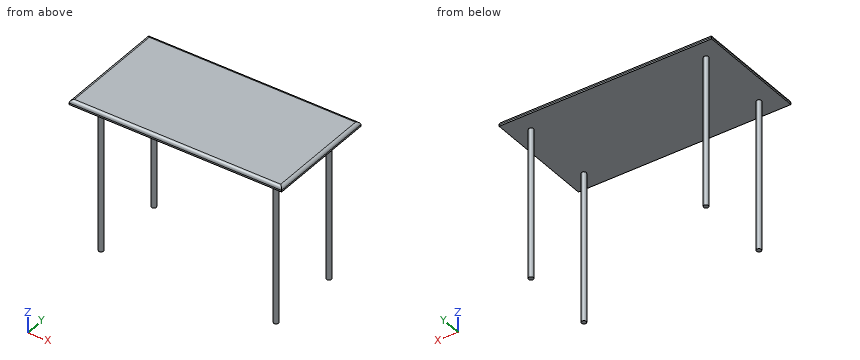
```python
from build123d import *

# Parameters (mm, degrees)
F0_R     = 9.525
F1_DEPTH = 609.6
F2_W     = 863.6
F2_H     = 457.2
F2_R     = 9.525
F3_DEPTH = 19.05
F4_R     = 12.7


with BuildPart() as f1:
    # F0 (on Top) → F1 (new body)
    with BuildSketch(Plane.XY):
        with Locations((9.933765, 11.337449)):
            Circle(F0_R)
        with Locations((9.933765, 316.137449)):
            Circle(F0_R)
        with Locations((721.133765, 11.337449)):
            Circle(F0_R)
        with Locations((721.133765, 316.137449)):
            Circle(F0_R)
    extrude(amount=F1_DEPTH)

    # F2 (on face) → F3 (join)
    with BuildSketch(Plane.XY.offset(609.6)):
        with Locations((365.305165, 163.966049)):
            Rectangle(F2_W, F2_H)
        with Locations((9.933765, 11.337449)):
            Circle(F2_R, mode=Mode.SUBTRACT)
        with Locations((9.933765, 11.337449)):
            Circle(F2_R)
    extrude(amount=F3_DEPTH)

    # F4
    f4_edges = [f1.edges().sort_by_distance(p)[0] for p in [
        (797.105165, 163.966049, 628.65),
        (365.305165, 392.566049, 628.65),
        (-66.494835, 163.966049, 628.65),
        (365.305165, -64.633951, 628.65),
    ]]
    fillet(f4_edges, radius=F4_R)


solid = f1.part
```
Can you work these out from the model? Positions are in its coordinate system, mm. Give positions to 0.01 mm unless a question says otherwise; leave off trailing zeros. Order: outer loops, then holes, each group sorted by start corner. A loop starts at its lowest first (then second) coordinate and runs counter-clockwise, first axis right, second up. Notation, with made-up numbers: M -1.75,-20 L 13.25,-20 A26 cw 13.25,15 Z; hole C 14.5,89 d7. An arc over 180 degrees is marked long. One line per item, written item: value.
1) I want a section at C-C, the plane z = 368.5. List the corners of the cut face in (x, y) for me (3 decimals), plus the area to 3 significant figures.
Answer sheet:
outline: C 9.934,11.337 d19.05; C 9.934,316.137 d19.05; C 721.134,11.337 d19.05; C 721.134,316.137 d19.05
area: 1,140 mm^2
2) I want a section at A-A, the plane x = 309.5. List the corners of the cut face in (y, z) for me.
Answer sheet:
outline: M -64.63,609.6 L 392.57,609.6 L 392.57,615.95 A12.7 ccw 379.87,628.65 L -51.93,628.65 A12.7 ccw -64.63,615.95 Z
3) I want a section at B-B, the plane y = 35. List the corners of the cut face in (x, z) for me.
Answer sheet:
outline: M -66.49,609.6 L 797.11,609.6 L 797.11,615.95 A12.7 ccw 784.41,628.65 L -53.79,628.65 A12.7 ccw -66.49,615.95 Z
4) Please list where these lines run through material, in increasing order: line 1 along X through (y, z) = (316.5, 441); line 2 along Z through (x, y) = (-11.5, 283.5); line 3 along X through (y, z) = (16, 534.5).
Answer sheet:
line 1: x = 0.42 to 19.45, 711.62 to 730.65
line 2: z = 609.6 to 628.65
line 3: x = 1.63 to 18.24, 712.83 to 729.44
